Source: CAD feature listing. Evaluate the final solid. Frame: model axes, mm. Face numbers are marked on the shaded views. A direction names the side the tool comes from. Round coordinates to 2 decimals unless told otherwise and drop trailing zeros. Write each loop counter-clockwise with the first axis right and the second up, starting at its lowest first coordinate (ties: lowest second). Pieces come first, ordered by that corner, then holes.
from build123d import *

# Parameters (mm, degrees)
SKETCH_W     = 60
SKETCH_H     = 100
PAD_DEPTH    = 150
THICKNESS_T  = -1.6
SKETCH001_W  = 84
SKETCH001_H  = 40
POCKET_DEPTH = 1.6
PAD001_DEPTH = 10
SKETCH003_W  = 60
SKETCH003_H  = 102
SKETCH003_R  = 20
PAD002_DEPTH = 2
FILLET_R     = 25


with BuildPart() as part:
    # Sketch → Pad (new body)
    with BuildSketch(Plane.XY):
        Rectangle(SKETCH_W, SKETCH_H)
    extrude(amount=PAD_DEPTH)

    # Thickness
    thickness_openings = [part.faces().sort_by_distance(p)[0] for p in [
        (0, 0, 150),
    ]]
    offset(amount=THICKNESS_T, openings=thickness_openings)

    # Sketch001 (on Face4 of Thickness) → Pocket (cut)
    with BuildSketch(Plane(origin=(-30, 0, 0), x_dir=(0, -1, 0), z_dir=(-1, 0, 0))):
        with Locations((0, 28)):
            Rectangle(SKETCH001_W, SKETCH001_H)
    extrude(amount=-POCKET_DEPTH, mode=Mode.SUBTRACT)

    # Sketch002 (on Face6 of Pocket) → Pad001 (join)
    with BuildSketch(Plane(origin=(0, 50, 0), x_dir=(-1, 0, 0), z_dir=(0, 1, 0))):
        Polygon((-30, 102), (-30, 0), (30, 0), (30, 2), (-28, 2), (-28, 102), align=None)
    extrude(amount=PAD001_DEPTH)

    # Sketch003 (on Face19 of Pad001) → Pad002 (join)
    with BuildSketch(Plane(origin=(0, 60, 0), x_dir=(-1, 0, 0), z_dir=(0, 1, 0))):
        with Locations((0, 51)):
            Rectangle(SKETCH003_W, SKETCH003_H)
        with Locations((0, 75)):
            Circle(SKETCH003_R, mode=Mode.SUBTRACT)
        with Locations((0, 25)):
            Circle(SKETCH003_R, mode=Mode.SUBTRACT)
    extrude(amount=PAD002_DEPTH)

    # Fillet
    fillet_edges = [part.edges().sort_by_distance(p)[0] for p in [
        (-30, 61, 102),
    ]]
    fillet(fillet_edges, radius=FILLET_R)


solid = part.part
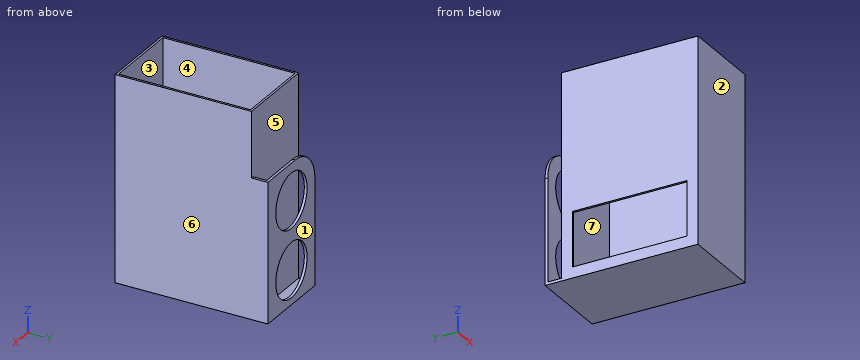
1) Section query D-D on z = 132.5. Return the cut outline in (x, y).
Taken from the geometry:
outline: (-30, -50) - (30, -50) - (30, 50) - (-30, 50) - close; hole (-28.4, -48.4) - (28.4, -48.4) - (28.4, 48.4) - (-28.4, 48.4) - close
2) Material intervals for line 1 (Y direction, x = -20, z = 9); line 2 (Z direction, x = 0, y = 61.15); line 3 (X direction, y = 3, z = 110), sorted ascending.
Taken from the geometry:
line 1: y = -50 to -48.4, 48.4 to 50, 60 to 62
line 2: z = 0 to 5, 45 to 55, 95 to 102
line 3: x = -30 to -28.4, 28.4 to 30
3) Section query C-C on x = 0. Return the cut outline in (y, z).
Taken from the geometry:
outline: (-50, 0) - (62, 0) - (62, 5) - (60, 5) - (60, 2) - (50, 2) - (50, 150) - (48.4, 150) - (48.4, 1.6) - (-48.4, 1.6) - (-48.4, 150) - (-50, 150) - close; (60, 45) - (62, 45) - (62, 55) - (60, 55) - close; (60, 95) - (62, 95) - (62, 102) - (60, 102) - close
4) Reachability of the marked faces 5, 6 and 7 from +Z, -Z, +X, -X, +Y, -Y: full face, straight path, thin tool, end or side. Return the list, or none.
Taken from the geometry:
face 5: +Z, -X
face 6: +Z, -Z, +X, +Y, -Y
face 7: +Z
5) Section query B-B on z = 67.5. Return the cut outline in (x, y).
Taken from the geometry:
outline: (-30, -50) - (30, -50) - (30, 62) - (18.54, 62) - (18.54, 60) - (28, 60) - (28, 50) - (-30, 50) - close; (-30, 60) - (-18.54, 60) - (-18.54, 62) - (-30, 62) - close; hole (-28.4, -48.4) - (28.4, -48.4) - (28.4, 48.4) - (-28.4, 48.4) - close
6) Section query A-A on y = -19.5. Return the cut outline in (x, z), then the cut area to 3 significant figures.
Taken from the geometry:
outline: (-30, 0) - (30, 0) - (30, 150) - (28.4, 150) - (28.4, 1.6) - (-28.4, 1.6) - (-28.4, 8) - (-30, 8) - close; (-30, 48) - (-28.4, 48) - (-28.4, 150) - (-30, 150) - close
area: 507 mm2
7) Pull-direction query (Y, two-part tool) for the marked faces 1, 2, 3 and 4; classes: released by +Y, released by -Y, zero draft, split by the parting line, or undercut.
Taken from the geometry:
face 1: released by +Y
face 2: released by -Y
face 3: undercut
face 4: undercut
8) Contact query for flat-ended pins moving along their axis: P1, Ø3, axis at x = 7.5, y = 55.5, coming from the +Z side; P2, Ø8, axis at x = 5.5, y = 44.5, coming from the -Z side; P3, Ø6, axis at y = -21, z = 31, coming from the -X side. Output: stop coordinate, or through.
Taken from the geometry:
P1: stops at z = 2
P2: stops at z = 0
P3: stops at x = 28.4
